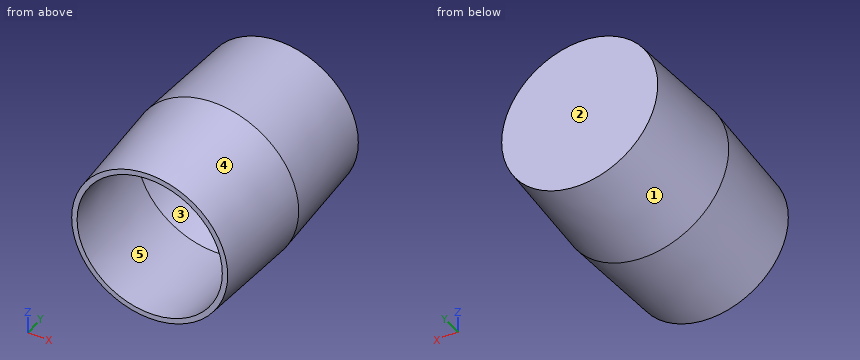
```python
from build123d import *

# Parameters (mm, degrees)
F0_R     = 39.3007161627
F1_DEPTH = 50.8
F1_TAPER = 3
F2_T     = -2.54


with BuildPart() as f1:
    # F0 (on Front) → F1 (new body, symmetric)
    with BuildSketch(Plane.XZ):
        Circle(F0_R)
    extrude(amount=F1_DEPTH, both=True, taper=F1_TAPER)

    # F2
    f2_openings = [f1.faces().sort_by_distance(p)[0] for p in [
        (0, -50.8, 0),
    ]]
    offset(amount=F2_T, openings=f2_openings, kind=Kind.INTERSECTION)


solid = f1.part
```
Part model, mm, in its own coordinate system. Face numbers are marked on the shaded views. A direction names the side the tool comes from. Round coordinates to 2 decimals unless told otherwise and drop trailing zeros. Loops run counter-clockwise (first coordinate to the right, second up) from the corner with the lowest first, then second, coordinate; pieces in that order, holes last.
Item 1: 3-axis set-ups, long thin cutter, end or side, ignore diameter. For the marked faces 4 and 5: which of +Z, -Z, +X, -X, +Y, -Y reach the whole face in a straight line?
Item 2: Mould opens along X. For the marked faces 1, 2 and 3 say: +X half, -X half, draft (parallel to the pull), parting line (faces both ways), or undercut.
Item 3: Cut at B-B, the plane y = -28. Give the cut face in (x, z).
Item 4: Cut at C-C, the plane y = -5.5. Give the cut face in (x, z).
Item 5: Cut at A-A, the plane x = 0. Give the cut face in (y, z).
Item 6: Drop flat-ended pins along their axis: P1, Ø4, axis at x = 8, y = 34, coming from the -Z side; P2, Ø1.5, axis at y = -13, z = -20, coming from the +X side; P3, Ø6, axis at y = 21, z = -25.5, coming from the -X side. Give the stop position or say it passes through.
Item 7: Drill centre lines: line 1 (Y direction, x = -7, z = -9); line 2 (X direction, y = 10, z = 7); line 3 (Z direction, x = 13, y = 0.5). Where is each one in solid material? Low to high.
A:
1. face 4: -Y
1. face 5: none
2. face 1: parting line
2. face 2: draft
2. face 3: undercut
3. outline: circle Ø75.67 at (0, 0); hole circle Ø70.58 at (0, 0)
4. outline: circle Ø78.02 at (0, 0); hole circle Ø72.94 at (0, 0)
5. outline: (-50.8, -36.64) - (0, -39.3) - (50.8, -36.64) - (50.8, 36.64) - (0, 39.3) - (-50.8, 36.64) - (-50.8, 34.09) - (0, 36.76) - (48.26, 34.23) - (48.26, -34.23) - (0, -36.76) - (-50.8, -34.09) - close
6. P1: stops at z = -37.05
6. P2: stops at x = 33.48
6. P3: stops at x = -30.88
7. line 1: y = 48.26 to 50.8
7. line 2: x = -38.14 to -35.55, 35.55 to 38.14
7. line 3: z = -37.06 to -34.35, 34.35 to 37.06
